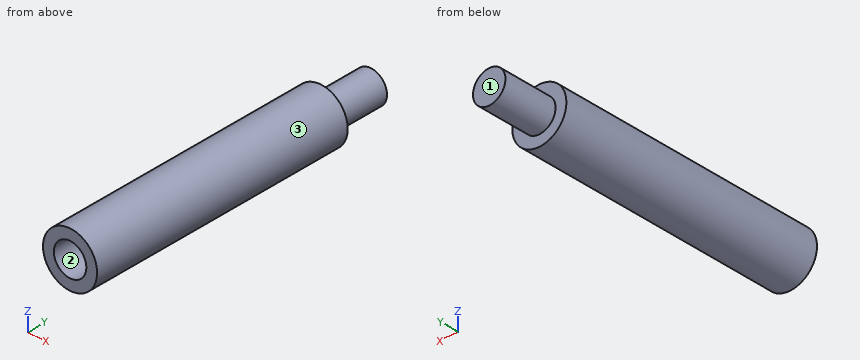
Autodesk Inventor part; units mm, degrees
ref_plane "YZ Plane" through (0, 0, 0) normal (1, 0, 0) x (0, 1, 0)
ref_plane "XZ Plane" through (0, 0, 0) normal (0, 1, 0) x (-1, 0, 0)
ref_plane "XY Plane" through (0, 0, 0) normal (0, 0, 1) x (1, 0, 0)
sketch "Sketch1" plane through (0, 0, 0) normal (0, 0, 1) x (1, 0, 0)
  line L0 (0, 24) -> (-1.5, 24)
  line L1 (-1.5, 24) -> (-1.5, 19)
  line L2 (-1.5, 19) -> (-2.5, 19)
  line L3 (-2.5, 19) -> (-2.5, -6)
  line L4 (-2.5, -6) -> (-1.5, -6)
  line L5 (-1.5, -6) -> (-1.5, 0)
  line L6 (-1.5, 0) -> (0, 0)
  line L7 (0, 0) -> (0, 24)
  dimension "d0" = 1.5
  dimension "d2" = 2.5
  dimension "d4" = 5
  dimension "d5" = 25
  dimension "d9" = 6
revolve "Revolution1" add sketch "Sketch1" angle 360 about axis through (0, 0, 0) along (0, 1, 0)
thread "Thread1"
thread "Thread2"
properties part number "Fitting-3" material "Brass"
Geometry check sheet. Reference: the model listing, model coordinates, mm. Face numbers are marked on the shaded views. Give positions to 0.01 mm unless a question says otherwise; leave off trailing zeros. Loops run counter-clockwise (first coordinate to the right, second up) from the corner with the lowest first, then second, coordinate; pieces in that order, holes last.
(1) Section check C-C on y = 12. Record the cut outline in (x, z).
From the geometry:
outline: circle Ø5 at (0, 0)
(2) Depth check by flat-ended pin: pin 1 Ø3 at (y, z) = (19.5, -2) entering from -X; pin 2 Ø0.9 at (x, z) = (0.5, -0.5) entering from -Y. Enter the tip coordinate at first touch or a pass-through.
From the geometry:
pin 1: stops at x = -2.43
pin 2: stops at y = 0
(3) Section check B-B on z = 0. Record the cut outline in (x, y).
From the geometry:
outline: (-2.5, -6) - (-1.5, -6) - (-1.5, 0) - (1.5, 0) - (1.5, -6) - (2.5, -6) - (2.5, 19) - (1.5, 19) - (1.5, 24) - (-1.5, 24) - (-1.5, 19) - (-2.5, 19) - close
(4) Section check A-A on x = 0. Record the cut outline in (y, z).
From the geometry:
outline: (-6, -2.5) - (19, -2.5) - (19, -1.5) - (24, -1.5) - (24, 1.5) - (19, 1.5) - (19, 2.5) - (-6, 2.5) - (-6, 1.5) - (0, 1.5) - (0, -1.5) - (-6, -1.5) - close
(5) Thickness scan on L1, parallel to Z at x = 0, y = -4; L2, parallel to Y at x = 0.05, z = 1.65; L3, parallel to Y at x = 0.55, z = -1.3. Record the ranges inside material, lowest first.
From the geometry:
L1: z = -2.5 to -1.5, 1.5 to 2.5
L2: y = -6 to 19
L3: y = 0 to 24
(6) Release check for a two-part mould opening along Z. For the marked faces 1, 2 and 3 record: released by +Z, released by -Z, zero draft, split by the parting line, or undercut.
From the geometry:
face 1: zero draft
face 2: undercut
face 3: split by the parting line
